Can you work these out from the drawing? Everything is in mm from the part's minimum corner. A direction names the side the tool comes from. Give positions to 0.01 mm unless a question says otherwise; leave off trailing zeros. Write each loop counter-clockwise with the first axis right and the second up, starting at its lowest first coordinate (ties: lowest second). Pieces come first, ordered by that corner, then holes. Notation, with made-up numbers: (76.25, -4) - (84.25, -4) arc R26 ccw to (84.25, 23) - close; hole circle Ø3 at (79, 8.5). An arc over 180 degrees is marked (long way). Use a Markdown table: item, result.
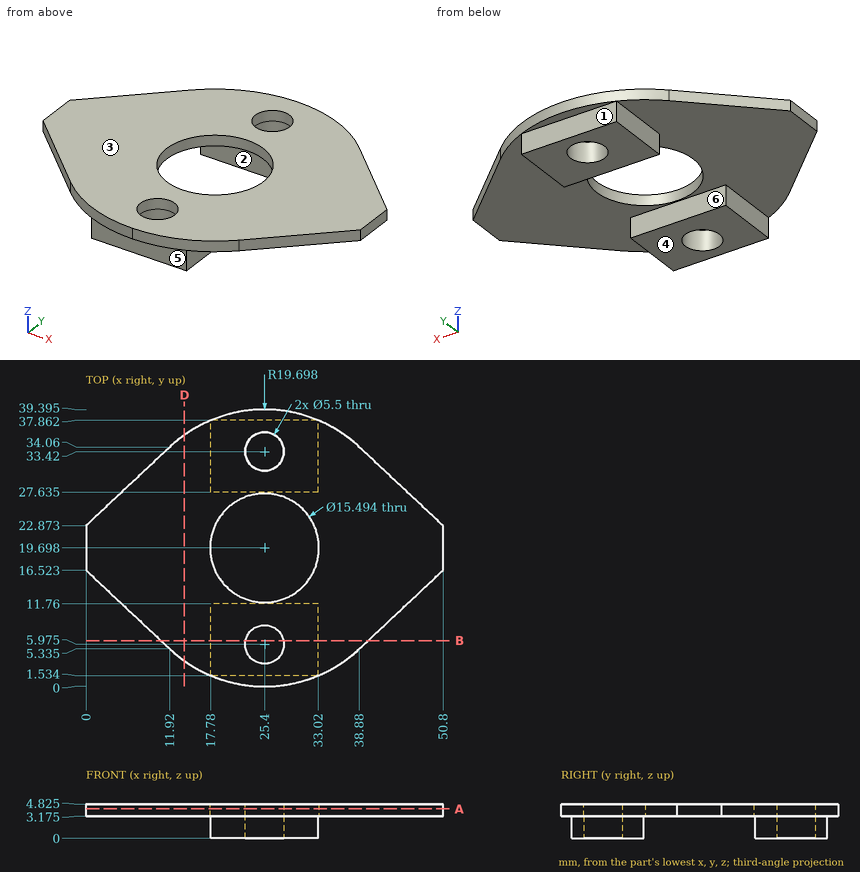
Item 1: Will these pins go through, and if not, where does the flat tip stop? pin 1 Ø1.6 at (y, z) = (31, 1.5) entering from -X; pin 2 Ø1 at (x, z) = (21.5, 1.5) entering from +Y; pin 3 Ø1.2 at (x, y) = (23, 38.5) entering from -Z (3 decimals).
Values:
| item | result |
|---|---|
| pin 1 | stops at x = 17.78 |
| pin 2 | stops at y = 37.86 |
| pin 3 | stops at z = 3.175 |
Item 2: If we section it at A-A, the plane z = 4.2: Count the separate pieces of the cut face and the enclosed holes in it, plus the area to 3 significant figures.
Values:
| item | result |
|---|---|
| separate pieces | 1 |
| enclosed holes | 3 |
| area | 1,150 mm2 |
Item 3: If we section it at D-D, the plane x = 14: Write out the boundary of the cut face in (y, z) (1 decimal).
Values:
| item | result |
|---|---|
| outline | (3.6, 3.2) - (35.8, 3.2) - (35.8, 4.8) - (3.6, 4.8) - close |
Item 4: I need wall thicknesses on line 1 along Y through (x, z) = (21.5, 2) (1 decimal); line 2 along Y through (x, z) = (25.4, 1.55) (1 decimal); line 3 along Y through (x, z) = (25, 1.3) (1 decimal). Which ranges of each line are inside material? Lowest first, please. Write a range as [from, to].
Values:
| item | result |
|---|---|
| line 1 | y = [1.5, 11.8], [27.6, 37.9] |
| line 2 | y = [1.5, 3.2], [8.7, 11.8], [27.6, 30.7], [36.2, 37.9] |
| line 3 | y = [1.5, 3.3], [8.7, 11.8], [27.6, 30.7], [36.1, 37.9] |
Item 5: If we section it at B-B, the plane y = 6.5: Write out the boundary of the cut face in (x, z) (1 decimal).
Values:
| item | result |
|---|---|
| outline | (10.7, 3.2) - (17.8, 3.2) - (17.8, 0) - (22.7, 0) - (22.7, 4.8) - (10.7, 4.8) - close; (28.1, 0) - (33, 0) - (33, 3.2) - (40.1, 3.2) - (40.1, 4.8) - (28.1, 4.8) - close |
Item 6: For the marked faces 4, 5 and 6, which set-ups out of +Z, -Z, +X, -X, +Y, -Y let a thin tool reach every point of the face, with its end or its side?
Values:
| item | result |
|---|---|
| face 4 | -Z, +X, -X, +Y, -Y |
| face 5 | -Z, +X, -X, -Y |
| face 6 | -Z, +X, -X |
Item 7: Thinking about a two-plate mould opening in Y: for the marked faces 1, 2 and 3, which applies, +Y half, -Y half, draft (parallel to the pull), parting line (faces both ways), or undercut?
Values:
| item | result |
|---|---|
| face 1 | +Y half |
| face 2 | undercut |
| face 3 | draft |
